Source: CAD feature listing. Evaluate the final solid. Frame: model axes, mm. Face numbers are marked on the shaded views. A direction names the side the tool comes from. Give positions to 0.01 mm unless a question says otherwise; leave off trailing zeros. Loops run counter-clockwise (first coordinate to the right, second up) from the corner with the lowest first, then second, coordinate; pieces in that order, holes last.
Autodesk Inventor part; units mm, degrees
ref_plane "YZ Plane" through (0, 0, 0) normal (1, 0, 0) x (0, 1, 0)
ref_plane "XZ Plane" through (0, 0, 0) normal (0, 1, 0) x (-1, 0, 0)
ref_plane "XY Plane" through (0, 0, 0) normal (0, 0, 1) x (1, 0, 0)
sketch "Sketch1" plane through (0, 0, 0) normal (0, 0, 1) x (1, 0, 0)
  line L0 (0, 0) -> (-1.6043, 0)
  line L1 (-1.6043, 0) -> (-2.0043, 0)
  line L2 (-2.0043, 0) -> (-3.6043, 0)
  line L3 (0, 0) -> (0, -15)
  line L4 (0, -15) -> (-3.6043, -15)
  line L5 (-3.6043, -15) -> (-3.6043, 0)
  line L6 (0, 0) -> (0, 18.6)
  line L7 (0, 18.6) -> (-3.6043, 18.6)
  line L8 (-3.6043, 18.6) -> (-3.6043, 0)
  line L9 (-2.0043, 0) -> (-2.0043, -15)
  line L10 (-2.0043, 0.2824) -> (-2.0043, 18.6)
  line L11 (0, -15) -> (49.6, -15)
  line L12 (49.6, -15) -> (50, -15)
  line L13 (50, -15) -> (51.6, -15)
  line L14 (51.6, -15) -> (51.6, 18.6)
  line L15 (51.6, 18.6) -> (50, 18.6)
  line L16 (50, 18.6) -> (50, -15)
  line L17 (50, 18.6) -> (-2.0043, 18.6)
  dimension "d0" = 0.4
  dimension "d1" = 1.6
  dimension "d2" = 15
  dimension "d4" = 49.6
  dimension "d5" = 0.4
  dimension "d6" = 1.6
extrude "Extrusion1" add sketch "Sketch1" along normal blind 1.6
sketch "Sketch2" plane through (0, 0, 0) normal (0, 0, -1) x (-1, 0, 0)
  line L0 (3.6043, 18.6) -> (3.6043, -15)
  line L1 (3.6043, 18.6) -> (2.0043, 18.6)
  line L2 (-51.6, 18.6) -> (3.6043, 18.6)
  line L3 (2.0043, 18.6) -> (2.0043, -15)
  line L4 (3.6043, -15) -> (-51.6, -15)
  line L5 (-51.6, -15) -> (-51.6, 18.6)
  line L6 (-51.6, 18.6) -> (-50, 18.6)
  line L7 (-50, 18.6) -> (-50, -15)
  line L8 (-51.6, 18.6) -> (-50, 18.6)
  line L9 (-51.6, -15) -> (-50, -15)
  line L10 (2.0043, 18.6) -> (3.6043, 18.6)
  line L11 (3.6043, -15) -> (2.0043, -15)
  point P0 (0, 0)
  dimension "d9" = 1.6
  dimension "d10" = 1.6
extrude "Extrusion2" add sketch "Sketch2" along normal blind 14.6 contours L0 L4 L3 L1 | L7 L4 L5 L2
sketch "Sketch3" plane through (-3.6043, -15, 1.6) normal (-1, 0, 0) x (0, 0, 1)
  line L0 (-16.2, 0) -> (0, 0)
  line L1 (0, 0) -> (0, 5)
  line L2 (0, 33.6) -> (0, 0)
  line L3 (0, 0) -> (-6.6, 0)
  line L4 (-1.6, 0) -> (-16.2, 0)
  line L5 (-6.6, 0) -> (-6.6, 5)
  circle A0 centre (-6.6, 5) radius 2.15
  point P0 (-1.6, 15)
  dimension "d13" = 5
  dimension "d14" = 6.6
  dimension "d15" = 4.3
extrude "Extrusion3" cut sketch "Sketch3" against normal blind 68.6
sketch "Sketch4" plane through (0, 0, 1.6) normal (0, 0, 1) x (1, 0, 0)
  line L0 (19.036, -6.8706) -> (33.9718, -6.8706)
  line L1 (33.9718, -6.8706) -> (33.9718, -8.566)
  line L2 (33.9718, -8.566) -> (19.036, -8.566)
  line L3 (19.036, -8.566) -> (19.036, -6.8706)
  point P0 (0, 0)
extrude "Extrusion4" cut sketch "Sketch4" against normal blind 68.6
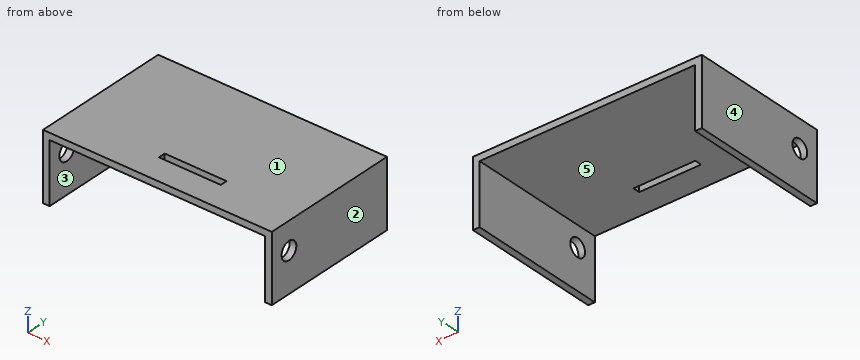
(1) Section B-B, the plane y = -10. Return the cut outline in (x, z), then the cut area to 3 significant figures.
A:
outline: (-3.6, -14.6) - (-2, -14.6) - (-2, -7.15) - (-3.6, -7.15) - close; (-3.6, -2.85) - (-2, -2.85) - (-2, 0) - (50, 0) - (50, -2.85) - (51.6, -2.85) - (51.6, 1.6) - (-3.6, 1.6) - close; (50, -14.6) - (51.6, -14.6) - (51.6, -7.15) - (50, -7.15) - close
area: 121 mm2
(2) Ray query, line 1 along Y through (x, z) = (-3.05, -5); line 2 along X through (y, z) = (11, -2.75); line 3 along Z through (x, y) = (50.7, -10). Return the intervals inside material, ascending.
A:
line 1: y = -15 to -12.15, -7.85 to 18.6
line 2: x = -3.6 to -2, 50 to 51.6
line 3: z = -14.6 to -7.15, -2.85 to 1.6
(3) Section A-A, the plane z = -13.25. Return the cut outline in (x, y), then the cut area to 3 significant figures.
A:
outline: (-3.6, -15) - (-2, -15) - (-2, 18.6) - (-3.6, 18.6) - close; (50, -15) - (51.6, -15) - (51.6, 18.6) - (50, 18.6) - close
area: 108 mm2
(4) Reachability of the marked faces 4 and 5 from +Z, -Z, +X, -X, +Y, -Y: full face, straight path, thin tool, end or side. Return the list, or none.
A:
face 4: +Z, -Z, -X, +Y, -Y
face 5: -Z, +Y, -Y
(5) Mould query, pull axis X, two halves, no side actions, for the marked faces 1, 2 and 3. Classes: pulls with the +X half, pulls with the -X half, needs draft (parallel to the pull), parting line crosses it, or undercut.
A:
face 1: needs draft
face 2: pulls with the +X half
face 3: undercut
(6) First-contact query: pin 1 (17 mm diameter, centred on x = 30, y = 6.5, fed in from -Z); pin 2 (2.5 mm diameter, centred on y = -10, z = -5, fed in from +X). Flat tips, straight axial feed; report the tip coordinate or a pass-through.
A:
pin 1: stops at z = 0
pin 2: passes through
(7) Section C-C, the plane x = 28. Return the cut outline in (y, z), then the cut area to 3 significant figures.
A:
outline: (-15, 0) - (-8.57, 0) - (-8.57, 1.6) - (-15, 1.6) - close; (-6.87, 0) - (18.6, 0) - (18.6, 1.6) - (-6.87, 1.6) - close
area: 51.0 mm2
(8) Section D-D, the plane z = -5. Return the cut outline in (x, y), then the cut area to 3 significant figures.
A:
outline: (-3.6, -15) - (-2, -15) - (-2, -12.15) - (-3.6, -12.15) - close; (-3.6, -7.85) - (-2, -7.85) - (-2, 18.6) - (-3.6, 18.6) - close; (50, -15) - (51.6, -15) - (51.6, -12.15) - (50, -12.15) - close; (50, -7.85) - (51.6, -7.85) - (51.6, 18.6) - (50, 18.6) - close
area: 93.8 mm2
